```python
from build123d import *

# Parameters (mm, degrees)
BOSS_EXTRUDE1_DEPTH = 25.4
SKETCH2_R           = 2.286
CUT_EXTRUDE1_DEPTH  = 190.072249682
SKETCH3_R           = 1.905
CUT_EXTRUDE2_DEPTH  = 20.32
SKETCH4_R           = 34.29
CUT_EXTRUDE3_DEPTH  = 63.5
CUT_EXTRUDE4_DEPTH  = 7.62
CUT_EXTRUDE5_DEPTH  = 190.072249682
CUT_EXTRUDE6_DEPTH  = 157.48
FILLET1_R           = 7.62


with BuildPart() as part:
    # Sketch1 → Boss-Extrude1 (new, symmetric)
    with BuildSketch(Plane.XY):
        Polygon((0, 0), (0, 63.5), (-25.4, 63.5), (-25.4, 82.55), (0, 82.55), (0, 173.99), (-25.4, 173.99), (-25.4, 180.34), (25.4, 180.34), (50.8, 0), align=None)
    extrude(amount=BOSS_EXTRUDE1_DEPTH, both=True)

    # Sketch2 → Cut-Extrude1 (cut, through all)
    with BuildSketch(Plane.XZ):
        with Locations((10.16, -11.43)):
            Circle(SKETCH2_R)
        with Locations((19.685, 0)):
            Circle(SKETCH2_R)
        with Locations((10.16, 11.43)):
            Circle(SKETCH2_R)
        with Locations((45.72, -6.35)):
            Circle(SKETCH2_R)
        with Locations((45.72, 6.35)):
            Circle(SKETCH2_R)
    extrude(amount=-CUT_EXTRUDE1_DEPTH, mode=Mode.SUBTRACT)

    # Sketch3 → Cut-Extrude2 (cut)
    with BuildSketch(Plane.XZ.offset(-63.5)):
        with Locations(Location((-12.7, -19.05, 0), (0, 0, 270))):
            Circle(SKETCH3_R)
        with Locations(Location((-12.7, 19.05, 0), (0, 0, 270))):
            Circle(SKETCH3_R)
    extrude(amount=-CUT_EXTRUDE2_DEPTH, mode=Mode.SUBTRACT)

    # Sketch4 → Cut-Extrude3 (cut)
    with BuildSketch(Plane.XZ):
        with Locations((-31.75, 0)):
            Circle(SKETCH4_R)
    extrude(amount=-CUT_EXTRUDE3_DEPTH, mode=Mode.SUBTRACT)

    # Sketch5 → Cut-Extrude4 (cut)
    with BuildSketch(Plane.XZ):
        with BuildLine():
            Line((29.567845881, -25.773285055), (18.829761526, -54.242627064))
            ThreePointArc((18.829761526, -54.242627064), (8.19263059, -59.053187889), (3.382069764, -48.416056953))
            Line((3.382069764, -48.416056953), (14.120154119, -19.946714945))
            ThreePointArc((14.120154119, -19.946714945), (24.757285055, -15.136154119), (29.567845881, -25.773285055))
        make_face()
        with BuildLine():
            Line((29.567845881, 25.773285055), (18.829761526, 54.242627064))
            ThreePointArc((18.829761526, 54.242627064), (8.19263059, 59.053187889), (3.382069764, 48.416056953))
            Line((3.382069764, 48.416056953), (14.120154119, 19.946714945))
            ThreePointArc((14.120154119, 19.946714945), (24.757285055, 15.136154119), (29.567845881, 25.773285055))
        make_face()
    extrude(amount=-CUT_EXTRUDE4_DEPTH, mode=Mode.SUBTRACT)

    # Sketch6 → Cut-Extrude5 (cut, through all)
    with BuildSketch(Plane.XZ):
        Polygon((50.8, 25.4), (50.8, 12.7), (34.29, 25.4), align=None)
        Polygon((34.29, -25.4), (50.8, -25.4), (50.8, -12.7), align=None)
    extrude(amount=-CUT_EXTRUDE5_DEPTH, mode=Mode.SUBTRACT)

    # Sketch7 → Cut-Extrude6 (cut)
    with BuildSketch(Plane(origin=(0, 180.34, 0), x_dir=(1, 0, 0), z_dir=(0, 1, 0))):
        with BuildLine():
            Line((0, 31.75), (50.8, 31.75))
            Line((50.8, 31.75), (50.8, -31.75))
            Line((50.8, -31.75), (0, -31.75))
            ThreePointArc((0, -31.75), (31.75, 0), (0, 31.75))
        make_face()
    extrude(amount=-CUT_EXTRUDE6_DEPTH, mode=Mode.SUBTRACT)

    # Fillet1
    fillet1_edges = [part.edges().sort_by_distance(p)[0] for p in [
        (31.75, 22.86, 0),
    ]]
    fillet(fillet1_edges, radius=FILLET1_R)


solid = part.part
```
Check sheet for the modelled part. Datum: model origin and axes. Units: mm. A direction names the side the tool comes from. Round coordinates to 2 decimals unless told otherwise and drop trailing zeros. Order: outer loops, then holes, each group sorted by start corner. A loop starts at its lowest first (then second) coordinate and runs counter-clockwise, first axis right, second up. Notation, with made-up numbers: (2.5, 18.5) - (22.5, 18.5) arc R3 ccw to (22.5, 22.5) - close; hole circle Ø11 at (54, 77). An arc over 180 degrees is marked (long way). Write item = value, one per line.
Q1. Section check C-C (x = -3.5). Record the boundary of the cut face in (y, z).
Computed:
outline = (63.5, -25.4) - (82.55, -25.4) - (82.55, 25.4) - (63.5, 25.4) - close; (173.99, -25.4) - (180.34, -25.4) - (180.34, 25.4) - (173.99, 25.4) - close
Q2. Section check B-B (y = 41). State how many separate pieces and enclosed holes the cut face has, and give its area (3 significant figures).
Computed:
separate_pieces = 1
enclosed_holes = 3
area = 1,330 mm^2
Q3. Go/stop test with flat-tipped pins: pin 1 (5.5 mm diameter, centred on x = 18.5, z = 22.5, fed in from -Y); pin 2 (5 mm diameter, centred on x = -12.7, z = 19.05, fed in from -Y); pin 3 (12 mm diameter, centred on y = 52, z = -1, fed in from -X). Record where each tip stops, or that it passes through.
Computed:
pin_1 = 7.62
pin_2 = 63.5
pin_3 = 1.82
Q4. Tool access check on faces 4 (the face through (31.747, 89.808, 0.412)), 5 (the face through (13.08, 3.76, 22.71)), 6 (the face through (13.08, 3.76, -22.71)). Record the directions out of +Z, -Z, +X, -X, +Y, -Y that give a thin tool (end or side, any length) a straight path to the whole face; none if there is none.
Computed:
face_4 = +X, +Y
face_5 = +Z, -Y
face_6 = -Z, -Y
Q5. Section check A-A (z = 0). Record the boundary of the cut face in (x, y) (3 decimals), and give its area (3 significant figures).
Computed:
outline = (-25.4, 63.5) - (2.54, 63.5) - (2.54, 0) - (17.399, 0) - (17.399, 180.34) - (-25.4, 180.34) - (-25.4, 173.99) - (0, 173.99) - (0, 82.55) - (-25.4, 82.55) - close; (21.971, 0) - (50.8, 0) - (47.58, 22.86) - (39.37, 22.86) arc R7.62 cw to (31.75, 30.48) - (31.75, 135.255) - (25.4, 180.34) - (21.971, 180.34) - close
area = 5,650 mm^2
Q6. Draft check along Y on faces 1 (the face through (0, 31, 19)), 2 (the face through (-13, 173.99, 0)), 3 (the face through (21, 7.62, -21)). Enter one of: pulls with the +Y half, pulls with the -Y half, needs draft (parallel to the pull), parting line crosses it, or undercut.
Computed:
face_1 = needs draft
face_2 = undercut
face_3 = pulls with the -Y half
Q7. Thickness scan on line 1 along Z through (x, y) = (10.16, 45.5); line 2 along Y through (x, z) = (-18, 8); line 3 along X through (y, z) = (135, -1). Record the ranges inside material, lowest first.
Computed:
line_1 = -25.4 to -13.72, -9.14 to 9.14, 13.72 to 25.4
line_2 = 63.5 to 82.55, 173.99 to 180.34
line_3 = 0 to 17.63, 21.74 to 31.73
